Verification items for the finished model (mm, model axes). Face numbers are marked on the shaded views. A direction names the side the tool comes from. Give positions to 0.01 mm unless a question says otherwise; leave off trailing zeros. Loops run counter-clockwise (first coordinate to the right, second up) from the corner with the lowest first, then second, coordinate; pieces in that order, holes last. Notation, with made-up numbers: M -40,13 L -27,13 A26 cw -27,32 Z; hole C 84,55 d5. An arc over 180 degrees is marked long. Use a Markdown table: item, result.
from build123d import *

# Parameters (mm, degrees)
F0_W     = 13.3
F0_H     = 5.9
F1_DEPTH = 25
F2_W     = 3
F2_H     = 8
F3_DEPTH = 6
F4_SIZE  = 2


with BuildPart() as f1:
    # F0 (on Front) → F1 (new body)
    with BuildSketch(Plane.XZ):
        Rectangle(F0_W, F0_H)
    extrude(amount=F1_DEPTH)

    # F2 (on Front) → F3 (join)
    with BuildSketch(Plane.XZ):
        with Locations((-4, 4)):
            Rectangle(F2_W, F2_H)
        with Locations((4, 4)):
            Rectangle(F2_W, F2_H)
    extrude(amount=-F3_DEPTH)

    # F4
    f4_edges = [f1.edges().sort_by_distance(p)[0] for p in [
        (-4, 0, 8),
        (4, 0, 8),
        (4, 6, 0),
        (-4, 6, 0),
    ]]
    chamfer(f4_edges, length=F4_SIZE)


solid = f1.part
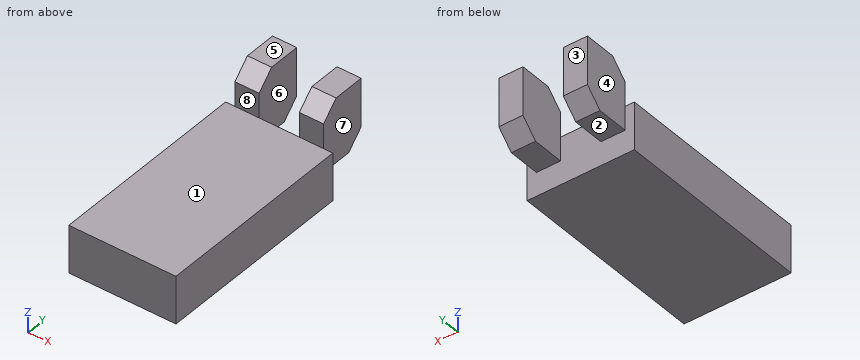
(1) Set-up check for the marked faces 1, 2, 3, 4 and 5: record each of +Z, -Z, +X, -X, +Y, -Y from which the full face is reachable in a straight line by a thin tool's end or side.
Results below:
| item | result |
|---|---|
| face 1 | +Z, +X, -X, -Y |
| face 2 | -Z, +X, -X, +Y |
| face 3 | +Z, -Z, +X, -X, +Y |
| face 4 | +Z, -Z, -X, +Y |
| face 5 | +Z, +X, -X, +Y, -Y |
(2) Draft check along X on the marked faces 6, 7 and 8. Enter one of: +X half, -X half, draft (parallel to the pull), parting line (faces both ways), or undercut.
Results below:
| item | result |
|---|---|
| face 6 | undercut |
| face 7 | +X half |
| face 8 | draft |
(3) Gauge pin test, flat ends, axial feed: P1, Ø0.9, axis at x = 4, y = 2, coming from the -Z side; P2, Ø6.5, axis at y = 4, z = 4, coming from the -X side; P3, Ø1.8, axis at y = 4.5, z = 4.5, coming from the +X side. Record the tip position at first contact, or that the pin passes through.
Results below:
| item | result |
|---|---|
| P1 | z = 0 |
| P2 | x = -5.5 |
| P3 | x = 5.5 |
(4) Cross-section at B-B on y = 3. Record the cut outline in (x, z), then the cut area to 3 significant figures.
Results below:
| item | result |
|---|---|
| outline | M -5.5,0 L -2.5,0 L -2.5,8 L -5.5,8 Z; M 2.5,0 L 5.5,0 L 5.5,8 L 2.5,8 Z |
| area | 48.0 mm^2 |
(5) Material ranges on line 1 (Z direction, x = 4.5, y = -7); line 2 (X direction, y = 2.5, z = 3.25); line 3 (Y direction, x = 2.25, z = -0.75), recorded low to high.
Results below:
| item | result |
|---|---|
| line 1 | -2.95 to 2.95 |
| line 2 | -5.5 to -2.5, 2.5 to 5.5 |
| line 3 | -25 to 0 |
(6) Cross-section at D-D on z = 1.5. Record the cut outline in (x, y), then the cut area to 4 significant figures.
Results below:
| item | result |
|---|---|
| outline | M -6.65,-25 L 6.65,-25 L 6.65,0 L 5.5,0 L 5.5,5.5 L 2.5,5.5 L 2.5,0 L -2.5,0 L -2.5,5.5 L -5.5,5.5 L -5.5,0 L -6.65,0 Z |
| area | 365.5 mm^2 |
(7) Cross-section at A-A on z = 5.25. Record the cut outline in (x, y), then the cut area to 3 significant figures.
Results below:
| item | result |
|---|---|
| outline | M -5.5,0 L -2.5,0 L -2.5,6 L -5.5,6 Z; M 2.5,0 L 5.5,0 L 5.5,6 L 2.5,6 Z |
| area | 36.0 mm^2 |
(8) Cross-section at C-C on x = -4.5. Record the cut outline in (y, z).
Results below:
| item | result |
|---|---|
| outline | M -25,-2.95 L 0,-2.95 L 0,0 L 4,0 L 6,2 L 6,8 L 2,8 L 0,6 L 0,2.95 L -25,2.95 Z |
